```python
from build123d import *

# Parameters (mm, degrees)
DOME2_FACE_RADIUS       = 12.7
DOME2_HEIGHT            = 5.08
CUT_EXTRUDE2_DEPTH      = 54.881536726
CUT_EXTRUDE2_DEPTH_BACK = 54.881536726
CHAMFER1_SIZE           = 0.762


with BuildPart() as part:
    # Sketch1 → Revolve1 (revolve)
    with BuildSketch(Plane.XY, mode=Mode.PRIVATE) as revolve1_sk:
        Polygon((0, 0), (0, 45.72), (-12.7, 45.72), (-12.7, 43.18), (-6.35, 43.18), (-6.35, 0), align=None)
    revolve(revolve1_sk.sketch.rotate(Axis((0, 0, 0), (0, 1, 0)), 270), axis=Axis((0, 0, 0), (0, 1, 0)))

    # Dome2: a dome of height H over a round flat face of radius A is a cap of a sphere of radius (A * A + H * H) / (2 * H)
    dome2_r = (DOME2_FACE_RADIUS * DOME2_FACE_RADIUS + DOME2_HEIGHT * DOME2_HEIGHT) / (2 * DOME2_HEIGHT)
    dome2_base = Plane((0, 45.72, 0), z_dir=(0, 1, 0))
    with Locations(dome2_base.offset(DOME2_HEIGHT - dome2_r)):
        dome2_ball = Sphere(dome2_r, mode=Mode.PRIVATE)
    add(split(dome2_ball, bisect_by=dome2_base, keep=Keep.TOP, mode=Mode.PRIVATE))

    # Sketch2 → Cut-Extrude2 (cut, two sides: drawn at the far end of the back side and taken through both)
    with BuildSketch(Plane.XY.offset(-CUT_EXTRUDE2_DEPTH_BACK)):
        Polygon((1.27, 46.99), (-1.27, 46.99), (-3.262213041, 54.425040289), (3.262213041, 54.425040289), align=None)
    extrude(amount=CUT_EXTRUDE2_DEPTH + CUT_EXTRUDE2_DEPTH_BACK, mode=Mode.SUBTRACT)

    # Chamfer1
    chamfer1_edges = [part.edges().sort_by_distance(p)[0] for p in [
        (0, 0, 6.35),
    ]]
    chamfer(chamfer1_edges, length=CHAMFER1_SIZE)


solid = part.part
```
Build history of the part. All positions in model axes, mm. A direction names the side the tool comes from. Give positions to 0.01 mm unless a question says otherwise; leave off trailing zeros. Loops run counter-clockwise (first coordinate to the right, second up) from the corner with the lowest first, then second, coordinate; pieces in that order, holes last. Notation, with made-up numbers: (-12, 89.5) -> (45, 89.5) arc R17 ccw to (45, 108.5) -> close; hole circle Ø3 at (78, -13). An arc over 180 degrees is marked (long way). One line per question, with ' | ' between items. Start each with the question number.
1) Cut at D-D (z = -7). Give the cut face in (x, y) (3 decimals).
2) Probe L1, parallel to X at y = 2, z = 1.75; L2, parallel to Y at x = 5.25, z = 1; L3, parallel to X at y = 29.5, z = -3.5. List the from-to ranges inside material, lowest first.
3) Cut at A-A (z = 0). Give the cut face in (x, y) (3 decimals).
4) Two-plate mould, pull along X, no slides. Class faces 4 (the flat face through (0, 0, 0)), 5 (the flat face through (1.66, 48.44, -0.16)), 6 (the cylindrical face through (3.86, 21.67, 5.04)): released by +X, released by -X, zero draft, split by the parting line, or undercut.
5) Cut at C-C (y = 33). Give the cut face in (x, z).
6) Cut at B-B (x = 0). Give the cut face in (y, z) (3 decimals), plus the area to 3 significant figures.
7) Pin check, flat tips, straight feed: pin 1 (2 mm diameter, centred on y = 8.5, z = 0, fed in from -X); pin 2 (1.5 mm diameter, centred on x = -0.5, y = 35, fed in from -Z); pin 3 (1 mm diameter, centred on x = 2, z = -10, fed in from +Y). Stop position of each tip, or through.
8) 3-axis set-ups, long thin cutter, end or side, ignore diameter. For faces 1 (the flat face through (-1.646, 48.392, -0.156)), 2 (the cylindrical face through (7.7, 44.4, 10.1)), 3 (the flat face through (-6, 43.18, -3)): which of +Z, -Z, +X, -X, +Y, -Y reach the whole face in a straight line?
Return value:
1) outline: (-10.597, 43.18) -> (10.597, 43.18) -> (10.597, 45.72) arc R17.033 ccw to (1.892, 49.312) -> (1.27, 46.99) -> (-1.27, 46.99) -> (-1.892, 49.312) arc R17.033 ccw to (-10.597, 45.72) -> close
2) L1: -6.1 to 6.1 | L2: 0 to 50.01 | L3: -5.3 to 5.3
3) outline: (-12.7, 43.18) -> (-6.35, 43.18) -> (-6.35, 0.762) -> (-5.588, 0) -> (5.588, 0) -> (6.35, 0.762) -> (6.35, 43.18) -> (12.7, 43.18) -> (12.7, 45.72) arc R18.415 ccw to (2.254, 50.662) -> (1.27, 46.99) -> (-1.27, 46.99) -> (-2.254, 50.662) arc R18.415 ccw to (-12.7, 45.72) -> close
4) face 4: zero draft | face 5: undercut | face 6: split by the parting line
5) outline: circle Ø12.7 at (0, 0)
6) outline: (0, -5.588) -> (0.762, -6.35) -> (43.18, -6.35) -> (43.18, -12.7) -> (45.72, -12.7) arc R18.415 ccw to (46.99, -11.216) -> (46.99, 11.216) arc R18.415 ccw to (45.72, 12.7) -> (43.18, 12.7) -> (43.18, 6.35) -> (0.762, 6.35) -> (0, 5.588) -> close | area: 643 mm^2
7) pin 1: x = -6.35 | pin 2: z = -6.35 | pin 3: y = 48.04
8) face 1: +Z, -Z, +Y | face 2: +Y, -Y | face 3: -Y
